```python
from build123d import *

# Parameters (mm, degrees)
F1_DEPTH = 5.08
F2_R     = 0.635


# Not quite as in the source:
# - a feature names something its author has since deleted; it is built from what else it names


with BuildPart() as f1:
    # F0 (on Top) → F1 (new body)
    with BuildSketch(Plane.XY):
        with BuildLine():
            Line((3.7253e-06, 50.8), (4.3267840925, 7.8043183677))
            ThreePointArc((4.3267840925, 7.8043183677), (5.4175944315, 4.8348440923), (7.8057635016, 2.7601650422))
            ThreePointArc((7.8057635016, 2.7601650422), (18.8061487686, 0.162150538), (29.8082212267, 2.753010822))
            ThreePointArc((29.8082212267, 2.753010822), (32.2000000346, 4.8294123123), (33.2912774596, 7.8028215671))
            Line((33.2912774596, 7.8028215671), (37.5920037253, 50.8))
            Line((37.5920037253, 50.8), (3.7253e-06, 50.8))
        make_face()
    extrude(amount=F1_DEPTH)

    # F2
    f2_edges = [f1.edges().sort_by_distance(p)[0] for p in [
        (18.806149, 0.162151, 5.08),
        (32.2, 4.829412, 5.08),
        (35.441641, 29.301411, 5.08),
        (2.163394, 29.302159, 5.08),
        (5.417594, 4.834844, 5.08),
    ]]
    fillet(f2_edges, radius=F2_R)


solid = f1.part
```
The model under review builds one solid part; all positions refer to its coordinate system, in mm. Round coordinates to 2 decimals unless told otherwise and drop trailing zeros. Loops run counter-clockwise (first coordinate to the right, second up) from the corner with the lowest first, then second, coordinate; pieces in that order, holes last. Notation, with made-up numbers: (-40, 60) - (-7, 60) arc R21 ccw to (-7, 83) - close; hole circle Ø2 at (21, 64.25). An arc over 180 degrees is marked (long way). Write each question's results on one line, items separated by ' | '. Start each with the question number.
Q1. Take a section at A-A on z = 2.3. Give the boundary of the cut face in (x, y).
Q2. Insertion check: P1, Ø2, axis at x = 21.5, y = 25, coming from the -Z side; P2, Ø1, axis at y = 17, z = 3.5, coming from the -X side. Each pin has a flat end and moves straight along its axis. Give the tip position at first contact, or say it passes through.
Q3. Wall thickness on line 1 along X through (y, z) = (40, 2.85); line 2 along X through (y, z) = (28, 4.05); line 3 along Y through (x, z) = (22.5, 0.5): over which ranges is each line inside the solid? List them lowest first. Write a range as [from, to].
Data:
1) outline: (0, 50.8) - (4.33, 7.8) arc R6.35 ccw to (7.81, 2.76) arc R24.62 ccw to (29.81, 2.75) arc R6.35 ccw to (33.29, 7.8) - (37.59, 50.8) - close
2) P1: stops at z = 0 | P2: stops at x = 3.35
3) line 1: x = [1.09, 36.51] | line 2: x = [2.29, 35.31] | line 3: y = [0.44, 50.8]
